Here's how the part is built. I have some questions about the finished solid (model axes, mm). A direction names the side the tool comes from. Coordinates: 2 decimals unless noted, no trailing zeros. Write each loop counter-clockwise with the first axis right and the second up, starting at its lowest first coordinate (ties: lowest second). Pieces come first, ordered by that corner, then holes. Notation, with made-up numbers: (51.25, 32.25) -> (56.25, 32.25) arc R26 ccw to (56.25, 65.25) -> close; hole circle Ø3 at (73.25, -28). An arc over 180 degrees is marked (long way). Put each result on its own line as item: value. Start each with the question number.
Item 1: For pin 1 (2 mm diameter, centred on y = 2, z = 4, fed in from -X); pin 2 (1.5 mm diameter, centred on y = 2, z = 3, fed in from +X), each with a flat end and sliding along its axis, tell me the tip position at first contact or that it passes through.
Item 2: On a 3-axis mill with a long thin cutter (end or side, diameter ignored), from which of +Z, -Z, +X, -X, +Y, -Y can I reach the whole of each face in a straight line? I mean faces 4 (the face through (0.02, 0.09, 0.47)), 5 (the face through (-0.76, -0.43, 7.62)). Say none if no direction works.
Item 3: I want a section at A-A, the plane z = 6.25. List the corners of the cut face in (x, y) for me.
Item 4: I need wall thicknesses on line 1 (X direction, y = 0.35, z = 9); line 2 (X direction, y = -2.6, z = 5.25); line 3 (X direction, y = -0.55, z = 7.75). Which ranges of each line are inside material? Lowest first, please. Write a range as [from, to].
Item 5: If we mould it in two halves opening along Y, with no side actions, what happens to faces 1 (the face through (0, -2, 0)), 2 (the face through (-0.75, 0.44, 7.62)), 3 (the face through (-3, 0, 5))? For each: released by +Y, released by -Y, zero draft, split by the parting line, or undercut.
from build123d import *

# Parameters (mm, degrees)
SKETCH_1_W          = 3
SKETCH_1_H          = 10
CUT_EXTRUDE_1_DEPTH = 3
CHAMFER_1_SIZE      = 0.100000121
CHAMFER_1_SIZE2     = 0.100000075
CHAMFER_2_SIZE      = 1.125833025
CHAMFER_2_SIZE2     = 1
CHAMFER_3_SIZE      = 0.500000325
CHAMFER_3_SIZE2     = 0.500000243


with BuildPart() as part:
    # 草图1 → 旋转1 (revolve)
    with BuildSketch(Plane(origin=(0, 0, 0), x_dir=(1, 0, 0), z_dir=(0, 1, 0))):
        with Locations((1.5, -5)):
            Rectangle(SKETCH_1_W, SKETCH_1_H)
    revolve(axis=Axis((0, 0, 0), (0, 0, 1)))

    # 草图2 → 切除-拉伸1 (cut)
    with BuildSketch(Plane.XY.offset(10)):
        Polygon((0.75, -1.299038106), (1.5, 0), (0.75, 1.299038106), (-0.75, 1.299038106), (-1.5, 0), (-0.75, -1.299038106), align=None)
    extrude(amount=-CUT_EXTRUDE_1_DEPTH, mode=Mode.SUBTRACT)

    # 草图3 → 切除-旋转1 (revolve, cut)
    with BuildSketch(Plane(origin=(0, 0, 0), x_dir=(1, 0, 0), z_dir=(0, 1, 0)), mode=Mode.PRIVATE) as cut_revolve_1_sk:
        Polygon((1.499999, 0), (0, 0), (0, -0.500000312), align=None)
    revolve(cut_revolve_1_sk.sketch.rotate(Axis((0, 0, -2.5e-05), (0, 0, 1)), 180), axis=Axis((0, 0, -2.5e-05), (0, 0, 1)), mode=Mode.SUBTRACT)

    # 倒角1
    chamfer_1_edges = [part.edges().sort_by_distance(p)[0] for p in [
        (-3, 0, 10),
    ]]
    chamfer_1_side = [part.faces().sort_by_distance(p)[0] for p in [
        (-3, 0, 5),
    ]]
    chamfer(chamfer_1_edges, length=CHAMFER_1_SIZE, length2=CHAMFER_1_SIZE2, reference=chamfer_1_side[0])

    # 倒角2
    chamfer_2_edges = [part.edges().sort_by_distance(p)[0] for p in [
        (0, -1.299038106, 7),
        (-1.125, -0.649519053, 7),
        (-1.125, 0.649519053, 7),
        (0, 1.299038106, 7),
        (1.125, 0.649519053, 7),
        (1.125, -0.649519053, 7),
    ]]
    chamfer_2_side = [part.faces().sort_by_distance(p)[0] for p in [
        (0, 0, 7),
    ]]
    chamfer(chamfer_2_edges, length=CHAMFER_2_SIZE, length2=CHAMFER_2_SIZE2, reference=chamfer_2_side[0])

    # 倒角3
    chamfer_3_edges = [part.edges().sort_by_distance(p)[0] for p in [
        (-3, 0, 0),
    ]]
    chamfer_3_side = [part.faces().sort_by_distance(p)[0] for p in [
        (-3, 0, 4.94999994),
    ]]
    chamfer(chamfer_3_edges, length=CHAMFER_3_SIZE, length2=CHAMFER_3_SIZE2, reference=chamfer_3_side[0])


solid = part.part
Calculated:
1. pin 1: stops at x = -2.83
1. pin 2: stops at x = 2.73
2. face 4: -Z
2. face 5: +Z
3. outline: circle Ø6 at (0, 0)
4. line 1: x = [-2.98, -1.3], [1.3, 2.98]
4. line 2: x = [-1.5, 1.5]
4. line 3: x = [-2.95, -0.86], [0.86, 2.95]
5. face 1: zero draft
5. face 2: undercut
5. face 3: split by the parting line
